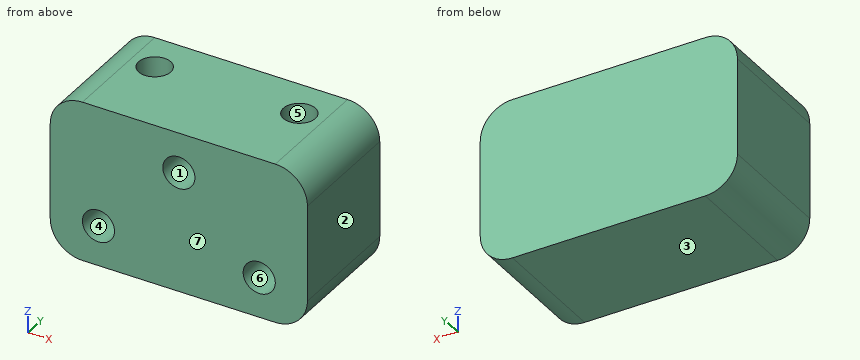
from build123d import *

# Parameters (mm, degrees)
BOSS_EXTRU_1_DEPTH      = 15
CONG_1_R                = 4
ESQUISSE2_R             = 2
ENL_V_MAT_EXTRU_1_DEPTH = 12
ESQUISSE3_R             = 2
ENL_V_MAT_EXTRU_2_DEPTH = 12


with BuildPart() as part:
    # Esquisse1 → Boss.-Extru.1 (new body)
    with BuildSketch(Plane(origin=(0, 0, 0), x_dir=(1, 0, 0), z_dir=(0, 1, 0))):
        Polygon((0, 0), (16, 0), (16, 20), (-16, 20), (-16, 0), align=None)
    extrude(amount=BOSS_EXTRU_1_DEPTH)

    # Congé1
    cong_1_edges = [part.edges().sort_by_distance(p)[0] for p in [
        (-16, 7.5, 0),
        (-16, 7.5, -20),
        (16, 7.5, -20),
        (16, 7.5, 0),
    ]]
    fillet(cong_1_edges, radius=CONG_1_R)

    # Esquisse2 → Enlèv. mat.-Extru.1 (cut)
    with BuildSketch(Plane.XZ):
        with Locations(Location((-10, -15, 0), (0, 0, 270))):
            Circle(ESQUISSE2_R)
        with Locations(Location((10, -15, 0), (0, 0, 270))):
            Circle(ESQUISSE2_R)
        with Locations(Location((0, -5, 0), (0, 0, 270))):
            Circle(ESQUISSE2_R)
    extrude(amount=-ENL_V_MAT_EXTRU_1_DEPTH, mode=Mode.SUBTRACT)

    # Esquisse3 → Enlèv. mat.-Extru.2 (cut)
    with BuildSketch(Plane.XY):
        with Locations((-9, 10)):
            Circle(ESQUISSE3_R)
        with Locations((9, 10)):
            Circle(ESQUISSE3_R)
    extrude(amount=-ENL_V_MAT_EXTRU_2_DEPTH, mode=Mode.SUBTRACT)


solid = part.part
The model under review builds one solid part; all positions refer to its coordinate system, in mm. Face numbers are marked on the shaded views. A direction names the side the tool comes from. Give positions to 0.01 mm unless a question says otherwise; leave off trailing zeros. Order: outer loops, then holes, each group sorted by start corner. A loop starts at its lowest first (then second) coordinate and runs counter-clockwise, first axis right, second up. Notation, with made-up numbers: M 32,64.25 L 83,64.25 A19 ccw 83,95.25 Z; hole C -8,27.25 d6. An arc over 180 degrees is marked long. Use one line per item in the form item = value. Start each with the question number.
Item 1: We need section B-B on z = -15. Give the boundary of the cut face in (x, y), plus the area to 3 significant figures.
Item 2: For the marked faces 5, 6 and 7, list the 3-axis set-ups (+Z, -Z, +X, -X, +Y, -Y) from which the entire face can be reached by the end or side of a thin tool; tool diameter is ignored.
Item 3: Insertion check: pin 1 Ø4.5 at (x, z) = (0, -4.5) entering from -Y. The pin has a flat end and moves straight along its axis. Give the tip position at first contact, or say it passes through.
Item 4: To check wall thickness, follow line 1 along X through (y, z) = (3, -15); line 2 along Y through (x, z) = (9, -4); line 3 along X through (y, z) = (6.25, -16.5). State the ranges of each line that lie inside material, in increasing order. Write a range as from..to.
Item 5: We need section D-D on y = 13.75. Give the boundary of the cut face in (x, z), plus the area to 3 significant figures.
Item 6: The part is to be moulded in two halves that separate along X. For the marked faces 1, 2, 3 and 4, say which applies: pulls with the +X half, pulls with the -X half, needs draft (parallel to the pull), parting line crosses it, or undercut.
Item 7: We need section C-C on x = 0. Give the boundary of the cut face in (y, z), plus the area to 3 significant figures.
Item 8: We need section A-A on y = 10. Give the boundary of the cut face in (x, z), plus the area to 3 significant figures.
Completed:
q1.outline = M -16,0 L -12,0 L -12,12 L -8,12 L -8,0 L 8,0 L 8,12 L 12,12 L 12,0 L 16,0 L 16,15 L -16,15 Z
q1.area = 384 mm²
q2.face_5 = +Z
q2.face_6 = -Y
q2.face_7 = +Z, -Z, +X, -X, -Y
q3.pin_1 = 0
q4.line_1 = -16..-12, -8..8, 12..16
q4.line_2 = 0..8, 12..15
q4.line_3 = -15.97..-11.32, -8.68..8.68, 11.32..15.97
q5.outline = M -16,-16 A4 ccw -12,-20 L 12,-20 A4 ccw 16,-16 L 16,-4 A4 ccw 12,0 L -12,0 A4 ccw -16,-4 Z
q5.area = 626 mm²
q6.face_1 = undercut
q6.face_2 = pulls with the +X half
q6.face_3 = needs draft
q6.face_4 = undercut
q7.outline = M 0,-20 L 15,-20 L 15,0 L 0,0 L 0,-3 L 12,-3 L 12,-7 L 0,-7 Z
q7.area = 252 mm²
q8.outline = M -16,-16 A4 ccw -12,-20 L 12,-20 A4 ccw 16,-16 L 16,-4 A4 ccw 12,0 L 11,0 L 11,-12 L 7,-12 L 7,0 L -7,0 L -7,-12 L -11,-12 L -11,0 L -12,0 A4 ccw -16,-4 Z; hole C -10,-15 d4; hole C 0,-5 d4; hole C 10,-15 d4
q8.area = 493 mm²
